```python
from build123d import *

# Parameters (mm, degrees)
F0_W     = 67.97842
F0_H     = 86.627372
F1_DEPTH = 30
F2_T     = -2.54
F3_R     = 5.08


with BuildPart() as f1:
    # F0 (on Front) → F1 (new body)
    with BuildSketch(Plane.XZ):
        Rectangle(F0_W, F0_H)
    extrude(amount=F1_DEPTH)

    # F2
    f2_openings = [f1.faces().sort_by_distance(p)[0] for p in [
        (0, -30, 0),
    ]]
    offset(amount=F2_T, openings=f2_openings)

    # F3
    f3_edges = [f1.edges().sort_by_distance(p)[0] for p in [
        (-33.98921, -15, 43.313686),
        (-33.98921, 0, 0),
        (33.98921, -15, 43.313686),
        (0, 0, 43.313686),
        (33.98921, 0, 0),
        (0, 0, -43.313686),
        (33.98921, -15, -43.313686),
        (-33.98921, -15, -43.313686),
    ]]
    fillet(f3_edges, radius=F3_R)


solid = f1.part
```
Input: part model. Units: mm. Frame: model coordinates. A direction names the side the tool comes from. Round coordinates to 2 decimals unless told otherwise and drop trailing zeros. Loops run counter-clockwise (first coordinate to the right, second up) from the corner with the lowest first, then second, coordinate; pieces in that order, holes last. Notation, with made-up numbers: M 88.25,-9.75 L 145.25,-9.75 A12 ccw 145.25,11.25 Z; hole C 51,-18 d9. An arc over 180 degrees is marked long. Answer in a Markdown table with one row per item. Add a question column.
1. Section C-C (z = -14). Output: boundary loops of the cut face in (x, y).
2. Section A-A (y = -28). Output: boundary loops of the cut face in (x, z).
3. Mould query, pull axis X, two halves, no side actions, for faces 1 (the face through (32.541, -17.714, 41.786)), 2 (the face through (0.4, -1.53, 41.87)), 3 (the face through (0, -16, -40.774)). Classes: released by +X, released by -X, zero draft, split by the parting line, or undercut.
4. Contact query for a flat-ended pin moving along its axis: pin 1 (4 mm diameter, centred on x = -19, z = -17, fed in from -Y). Output: stop coordinate, or through.
5. Section B-B (x = 22). Output: boundary loops of the cut face in (y, z), and give its area (3 significant figures).
6. Ray query, probe 1 along Z at (x, y) = (-19, -7.5); probe 2 along X at (y, z) = (-23.75, -37.5); probe 3 along Y at (x, z) = (-22.5, -35.5). Return the intervals inside material, ascending.
7. Set-up query: faces 4 (the face through (0, -16, 40.774)), 5 (the face through (-33, -30, 0)). Return all of +Z, -Z, +X, -X, +Y, -Y with unobstructed straight access to the full face (end or side cutting, diameter ignored); none if empty.
Values follow:
| question | item | result |
|---|---|---|
| 1 | outline | M -33.99,-30 L -31.45,-30 L -31.45,-2.54 L 31.45,-2.54 L 31.45,-30 L 33.99,-30 L 33.99,-5.08 A5.08 ccw 28.91,0 L -28.91,0 A5.08 ccw -33.99,-5.08 Z |
| 2 | outline | M -33.99,-38.23 A5.08 ccw -28.91,-43.31 L 28.91,-43.31 A5.08 ccw 33.99,-38.23 L 33.99,38.23 A5.08 ccw 28.91,43.31 L -28.91,43.31 A5.08 ccw -33.99,38.23 Z; hole M -31.45,-40.77 L 31.45,-40.77 L 31.45,40.77 L -31.45,40.77 Z |
| 3 | face 1 | released by +X |
| 3 | face 2 | zero draft |
| 3 | face 3 | undercut |
| 4 | pin 1 | y = -2.54 |
| 5 | outline | M -30,-43.31 L -5.08,-43.31 A5.08 ccw 0,-38.23 L 0,38.23 A5.08 ccw -5.08,43.31 L -30,43.31 L -30,40.77 L -2.54,40.77 L -2.54,-40.77 L -30,-40.77 Z |
| 5 | area | 348 mm^2 |
| 6 | probe 1 | -43.31 to -40.77, 40.77 to 43.31 |
| 6 | probe 2 | -33.99 to -31.45, 31.45 to 33.99 |
| 6 | probe 3 | -2.54 to 0 |
| 7 | face 4 | -Y |
| 7 | face 5 | +Z, -Z, +X, -X, -Y |
